```python
from build123d import *

# Parameters (mm, degrees)
SKETCH1_R           = 19
SKETCH1_R_2         = 13
BOSS_EXTRUDE1_DEPTH = 14
SKETCH3_R           = 21
SKETCH3_R_2         = 13
BOSS_EXTRUDE2_DEPTH = 1.5
FILLET1_R           = 1
CHAMFER2_SIZE       = 1


with BuildPart() as part:
    # Sketch1 → Boss-Extrude1 (new body)
    with BuildSketch(Plane.XY):
        Circle(SKETCH1_R)
        Circle(SKETCH1_R_2, mode=Mode.SUBTRACT)
    extrude(amount=BOSS_EXTRUDE1_DEPTH)

    # Sketch2 → Cut-Revolve1 (revolve, cut)
    with BuildSketch(Plane(origin=(0, 0, 0), x_dir=(1, 0, 0), z_dir=(0, 1, 0))):
        Polygon((-19, 0), (-17, -7), (-19, -14), align=None)
    revolve(axis=Axis((0, 0, 0), (0, 0, 1)), mode=Mode.SUBTRACT)

    # Sketch3 → Boss-Extrude2 (add)
    with BuildSketch(Plane(origin=(0, 0, 0), x_dir=(-1, 0, 0), z_dir=(0, 0, -1))):
        Circle(SKETCH3_R)
        with Locations(Location((0, 0, 0), (0, 0, 180))):
            Circle(SKETCH3_R_2, mode=Mode.SUBTRACT)
    boss_extrude2 = extrude(amount=-BOSS_EXTRUDE2_DEPTH)

    # Mirror1: Boss-Extrude2 across plane
    add(boss_extrude2.mirror(Plane.XY.offset(7)))

    # Fillet1
    fillet1_edges = [part.edges().sort_by_distance(p)[0] for p in [
        (17, 0, 7),
    ]]
    fillet(fillet1_edges, radius=FILLET1_R)

    # Chamfer2
    chamfer2_edges = [part.edges().sort_by_distance(p)[0] for p in [
        (-13, 0, 0),
        (-13, 0, 14),
    ]]
    chamfer(chamfer2_edges, length=CHAMFER2_SIZE)


solid = part.part
```
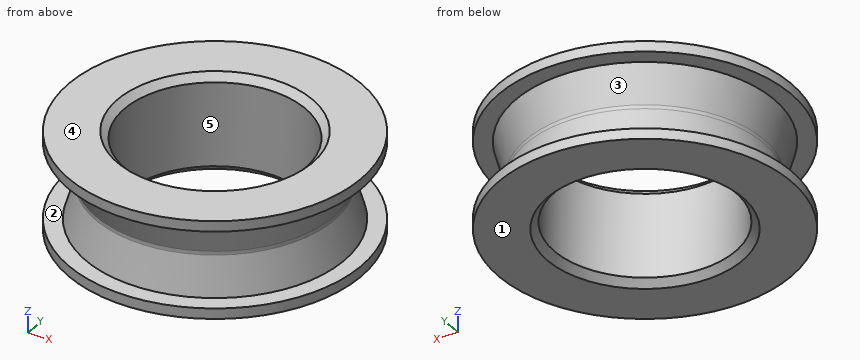
Build history of the part. All positions in model axes, mm. Face numbers are marked on the shaded views. A direction names the side the tool comes from. Give positions to 0.01 mm unless a question says otherwise; leave off trailing zeros. Return JSON: item names as keys, results as strings.
Q1. Two-plate mould, pull along Y, no slides. Class the marked faces 3, 4 and 5: pulls with the +Y half, pulls with the -Y half, needs draft (parallel to the pull), parting line crosses it, or undercut.
Answer list:
{"face 3": "parting line crosses it", "face 4": "needs draft", "face 5": "undercut"}
Q2. Wall check: probe 1 along Z at (x, y) = (-17, 8.5); probe 2 along X at (y, z) = (4.5, 13.25); probe 3 along Y at (x, z) = (-5.5, 8.25). Give the ranges that are in metal, low to high. Write a range as from..to.
Answer list:
{"probe 1": "z = 0..1.5, 12.5..14", "probe 2": "x = -20.51..-12.46, 12.46..20.51", "probe 3": "y = -16.46..-11.78, 11.78..16.46"}
Q3. 3-axis set-ups, long thin cutter, end or side, ignore diameter. For the marked faces 1 and 2: which of +Z, -Z, +X, -X, +Y, -Y reach the whole face in a straight line?
Answer list:
{"face 1": "-Z, +X, -X, +Y, -Y", "face 2": "none"}
Q4. Flat gauge pins, fed straight in: pin 1 (5 mm diameter, centred on x = -3, y = -11, fed in from -Z); pin 2 (4 mm diameter, centred on x = 0.5, z = 10, fed in from -Y); pin 3 (2 mm diameter, centred on x = -16, z = 7, fed in from -Y); pin 4 (3 mm diameter, centred on x = -11, y = -15.5, fed in from -Z). Where does each tip first touch, or does it go through?
Answer list:
{"pin 1": "stops at z = 0.1", "pin 2": "stops at y = -18.42", "pin 3": "stops at y = -8.1", "pin 4": "stops at z = 0"}
